Read the model definition and answer for the solid it produces. Units are mm, in the model's axes. A direction names the side the tool comes from. Give positions to 0.01 mm unless a question says otherwise; leave off trailing zeros. Loops run counter-clockwise (first coordinate to the right, second up) from the corner with the lowest first, then second, coordinate; pieces in that order, holes last. Notation, with made-up numbers: M -35,84.5 L -16,84.5 A26 ccw -16,100.5 Z; hole C 47,34 d1. An arc over 180 degrees is marked long. Return JSON: item names as keys, results as strings. Group by question number.
```python
from build123d import *

# Parameters (mm, degrees)
BOSS_EXTRUDE9_DEPTH      = 6.35
SKETCH4_W                = 3.261538064
SKETCH4_H                = 3.965348827
CUT_EXTRUDE2_DEPTH       = 26.406776986
SKETCH5_W                = 1.630769032
SKETCH5_H                = 1.267236454
CUT_EXTRUDE6_DEPTH       = 6.35
SKETCH6_W                = 1.630769032
SKETCH6_H                = 1.247570224
CUT_EXTRUDE7_DEPTH       = 6.477
CUT_EXTRUDE9_DEPTH       = 23.902768758
CUT_EXTRUDE9_DEPTH_BACK  = 23.902768758
SKETCH8_W                = 0.566855721
SKETCH8_H                = 1.002964872
CUT_EXTRUDE10_DEPTH      = 26.406776986
CUT_EXTRUDE10_DEPTH_BACK = 26.406776986
SKETCH9_W                = 0.508
SKETCH9_H                = 1.002964872
FILLET1_R                = 0.254
FILLET2_R                = 0.254
FILLET3_R                = 0.254
FILLET4_R                = 0.508
FILLET5_R                = 0.508
SKETCH11_W               = 5.19034067
SKETCH11_H               = 2.415254944
CUT_EXTRUDE11_DEPTH      = 30.316944626
FILLET6_R                = 1.143


with BuildPart() as part:
    # Sketch2 → Boss-Extrude9 (new, symmetric)
    with BuildSketch(Plane.XY):
        with BuildLine():
            Line((-5.471488307, -10.4902), (-4.36371454, -10.4902))
            ThreePointArc((-4.36371454, -10.4902), (-3.465688928, -10.862174388), (-3.09371454, -11.7602))
            Line((-3.09371454, -11.7602), (-3.09371454, -12.937827191))
            Line((-3.09371454, -12.937827191), (-10.566399977, -12.937827191))
            Line((-10.566399977, -12.937827191), (-10.566399977, -19.301956075))
            Line((-10.566399977, -19.301956075), (10.566399977, -19.301956075))
            Line((10.566399977, -19.301956075), (10.566399977, -12.937827191))
            Line((10.566399977, -12.937827191), (3.086674887, -12.937827191))
            Line((3.086674887, -12.937827191), (3.086674887, -11.7602))
            ThreePointArc((3.086674887, -11.7602), (3.458649275, -10.862174388), (4.356674887, -10.4902))
            Line((4.356674887, -10.4902), (5.476039751, -10.4902))
            Line((5.476039751, -10.4902), (5.476039751, -7.173536635))
            Line((5.476039751, -7.173536635), (3.650231899, -5.31386943))
            ThreePointArc((3.650231899, -5.31386943), (3.496357897, -5.285953607), (3.418648834, -5.421665813))
            ThreePointArc((3.418648834, -5.421665813), (0.00035136, -9.18188013), (-3.418715481, -5.422365367))
            ThreePointArc((-3.418715481, -5.422365367), (-3.496506609, -5.286643819), (-3.650404442, -5.314701882))
            Line((-3.650404442, -5.314701882), (-5.471488307, -7.173600332))
            Line((-5.471488307, -7.173600332), (-5.471488307, -10.4902))
        make_face()
    extrude(amount=BOSS_EXTRUDE9_DEPTH, both=True)

    # Sketch4 → Cut-Extrude2 (cut, through all)
    with BuildSketch(Plane.XY.offset(6.35)):
        with Locations((0, -11.95811765)):
            Rectangle(SKETCH4_W, SKETCH4_H)
    extrude(amount=-CUT_EXTRUDE2_DEPTH, mode=Mode.SUBTRACT)

    # Sketch5 → Cut-Extrude6 (cut, symmetric)
    with BuildSketch(Plane.XY.offset(6.35)):
        with Locations((-0.815384516, -9.341825009)):
            Rectangle(SKETCH5_W, SKETCH5_H)
    extrude(amount=CUT_EXTRUDE6_DEPTH, both=True, mode=Mode.SUBTRACT)

    # Sketch6 → Cut-Extrude7 (cut, symmetric)
    with BuildSketch(Plane(origin=(0, 0, -6.35), x_dir=(-1, 0, 0), z_dir=(0, 0, -1))):
        with Locations((-0.815384516, -9.351658124)):
            Rectangle(SKETCH6_W, SKETCH6_H)
    extrude(amount=CUT_EXTRUDE7_DEPTH, both=True, mode=Mode.SUBTRACT)

    # Sketch8 → Cut-Extrude9 (cut, two sides: drawn at the far end of the back side and taken through both)
    with BuildSketch(Plane.XY.offset(-CUT_EXTRUDE9_DEPTH_BACK)):
        with Locations((-3.377142401, -13.439309627)):
            Rectangle(SKETCH8_W, SKETCH8_H)
    extrude(amount=CUT_EXTRUDE9_DEPTH + CUT_EXTRUDE9_DEPTH_BACK, mode=Mode.SUBTRACT)

    # Sketch9 → Cut-Extrude10 (cut, two sides: drawn at the far end of the back side and taken through both)
    with BuildSketch(Plane.XY.offset(6.35).offset(-CUT_EXTRUDE10_DEPTH_BACK)):
        with Locations((3.340674887, -13.439309627)):
            Rectangle(SKETCH9_W, SKETCH9_H)
    extrude(amount=CUT_EXTRUDE10_DEPTH + CUT_EXTRUDE10_DEPTH_BACK, mode=Mode.SUBTRACT)

    # Fillet1
    fillet1_edges = [part.edges().sort_by_distance(p)[0] for p in [
        (-3.09371454, -13.940792063, 0),
    ]]
    fillet(fillet1_edges, radius=FILLET1_R)

    # Fillet2
    fillet2_edges = [part.edges().sort_by_distance(p)[0] for p in [
        (-3.660570261, -13.940792063, 0),
    ]]
    fillet(fillet2_edges, radius=FILLET2_R)

    # Fillet3
    fillet3_edges = [part.edges().sort_by_distance(p)[0] for p in [
        (3.594674887, -13.940792063, 0),
        (3.086674887, -13.940792063, 0),
        (1.630769032, -13.940792063, 0),
        (-1.630769032, -13.940792063, 0),
    ]]
    fillet(fillet3_edges, radius=FILLET3_R - 0.0001)  # a hair under: the kernel refuses the full size

    # Fillet4
    fillet4_edges = [part.edges().sort_by_distance(p)[0] for p in [
        (-10.566399977, -12.937827191, 0),
    ]]
    fillet(fillet4_edges, radius=FILLET4_R)

    # Fillet5
    fillet5_edges = [part.edges().sort_by_distance(p)[0] for p in [
        (-10.566399977, -19.301956075, 0),
        (10.566399977, -12.937827191, 0),
        (10.566399977, -19.301956075, 0),
    ]]
    fillet(fillet5_edges, radius=FILLET5_R)

    # Sketch11 → Cut-Extrude11 (cut, through all)
    with BuildSketch(Plane.ZY.offset(10.566399977)):
        with Locations((0, -16.044100378)):
            Rectangle(SKETCH11_W, SKETCH11_H)
    extrude(amount=-CUT_EXTRUDE11_DEPTH, mode=Mode.SUBTRACT)

    # Fillet6
    fillet6_edges = [part.edges().sort_by_distance(p)[0] for p in [
        (0, -14.836472906, 2.595170335),
        (0, -17.25172785, 2.595170335),
        (0, -17.25172785, -2.595170335),
        (0, -14.836472906, -2.595170335),
    ]]
    fillet(fillet6_edges, radius=FILLET6_R)


solid = part.part
```
1. Straight lines are drawn through the part: line 1 along Y through (x, z) = (7.5, -1); line 2 along X through (y, z) = (-9.75, -5.25); line 3 along Y through (x, z) = (1.5, 1). For each, find the intervals that lie inside material, in ascending order.
2. The mould has two halves that part along Y. Classify faces 5 (the flat face through (1.631, -11, 0)), 6 (the flat face through (0, -19.302, 0)), 7 (the flat face through (10.566, -18, 0)): +Y half, -Y half, draft (parallel to the pull), parting line (faces both ways), or undercut.
3. Find section D-D (y = -11.25). Write down the section's boundary in (x, z), and give its area (3 significant figures).
4. For faces 1 (the flat face through (5.476, -9, 0)), 2 (the cylindrical face through (0.15, -15.16, -2.25)), 3 (the cylindrical face through (-2.9, -7.59, 0.09)), 4 (the cylindrical face through (-3.48, -10.85, 0.09)), determine the directions among +Z, -Z, +X, -X, +Y, -Y from which every point of the face is accessible in a straight line to the end or side of a thin tool.
5. Find section A-A (x = 4). Write down the section's boundary in (y, z), and give its area (3 significant figures).
6. Find section B-B (y = -6.75). Write down the section's boundary in (x, z).
7. Find section C-C (x = -4.75). Write down the section's boundary in (y, z), and give its area (3 significant figures).
8. Flat-ended cylindrical pins translate along their axes: P1, Ø3, axis at x = 6, z = -2, coming from the +Y side; P2, Ø2, axis at y = -11, z = 0.5, coming from the -X side; P3, Ø0.8, axis at x = 0.5, z = 2, coming from the +Y side. Find the tip coordinate at first contact, or state that the pin passes through.
Result:
{
 "1": {"line 1": "y = -19.3 to -17.25, -14.84 to -12.94", "line 2": "x = -5.47 to 0, 1.63 to 5.48", "line 3": "y = -19.3 to -17.25, -14.84 to -13.91, -9.98 to -8.84"},
 "2": {"face 5": "undercut", "face 6": "-Y half", "face 7": "draft"},
 "3": {"outline": "M -3.2,-6.35 L -1.63,-6.35 L -1.63,6.35 L -3.2,6.35 Z; M 1.63,-6.35 L 3.19,-6.35 L 3.19,6.35 L 1.63,6.35 Z", "area": "39.8 mm2"},
 "4": {"face 1": "+Z, -Z, +X, +Y", "face 2": "+X, -X", "face 3": "+Z, -Z", "face 4": "+Z, -Z, -X"},
 "5": {"outline": "M -19.3,-6.35 L -12.94,-6.35 L -12.94,6.35 L -19.3,6.35 Z; M -10.54,-6.35 L -5.67,-6.35 L -5.67,6.35 L -10.54,6.35 Z; hole M -17.25,-1.45 A1.14 ccw -16.11,-2.6 L -15.98,-2.6 A1.14 ccw -14.84,-1.45 L -14.84,1.45 A1.14 ccw -15.98,2.6 L -16.11,2.6 A1.14 ccw -17.25,1.45 Z", "area": "131 mm2"},
 "6": {"outline": "M -5.06,-6.35 L -3.28,-6.35 L -3.28,6.35 L -5.06,6.35 Z; M 3.28,-6.35 L 5.06,-6.35 L 5.06,6.35 L 3.28,6.35 Z"},
 "7": {"outline": "M -19.3,-6.35 L -12.94,-6.35 L -12.94,6.35 L -19.3,6.35 Z; M -10.49,-6.35 L -6.44,-6.35 L -6.44,6.35 L -10.49,6.35 Z; hole M -17.25,-1.45 A1.14 ccw -16.11,-2.6 L -15.98,-2.6 A1.14 ccw -14.84,-1.45 L -14.84,1.45 A1.14 ccw -15.98,2.6 L -16.11,2.6 A1.14 ccw -17.25,1.45 Z", "area": "121 mm2"},
 "8": {"P1": "stops at y = -6.18", "P2": "stops at x = -5.47", "P3": "stops at y = -9.06"}
}
